Answer from the drawing. Dimensions are ordinates in mm from the lowest x, y and z of the part. Give positions to 0.01 mm unless a question says otherwise; leave off trailing zeros. Loops run counter-clockwise (first coordinate to the right, second up) from the corner with the lowest first, then second, coordinate; pieces in that order, holes last. Notation, with made-up numbers: (6.5, -12.5) - (31.5, -12.5) arc R28 ccw to (31.5, 7.5) - close; hole circle Ø8 at (75, 83.5). An arc over 180 degrees is marked (long way). Answer as CSV lines item,"result". Start each with the question number.
1) Find the intervals of material crossed by line 1 along Y through (x, z) = (0.6, 5) (1 decimal); line 2 along Z through (x, y) = (0.25, 4.25) (1 decimal); line 3 along Z through (x, y) = (0.1, 4.5) (1 decimal), in increasing order.
2) A cutting plane is placed at C-C (x = 0.1). Determine the outline of the cut face in (y, z) (1 decimal).
3) For a pull along Z with two mould halves and no side action, classify the marked faces 1, 2 and 3 as pulls with the +Z half, pulls with the -Z half, needs draft (parallel to the pull), parting line crosses it, or undercut.
4) A flat-ended cylindrical pin translates along its axis: pin 1 (1.9 mm diameter, centred on y = 3.96, z = 3.96, fed in from -X). Find the tip coordinate at first contact, or state that the pin passes through.
5) A cutting plane is placed at A-A (z = 4.75). Determine the outline of the cut face in (x, y) (1 decimal).
6) A cutting plane is placed at B-B (y = 4.5). Determine the outline of the cut face in (x, z).
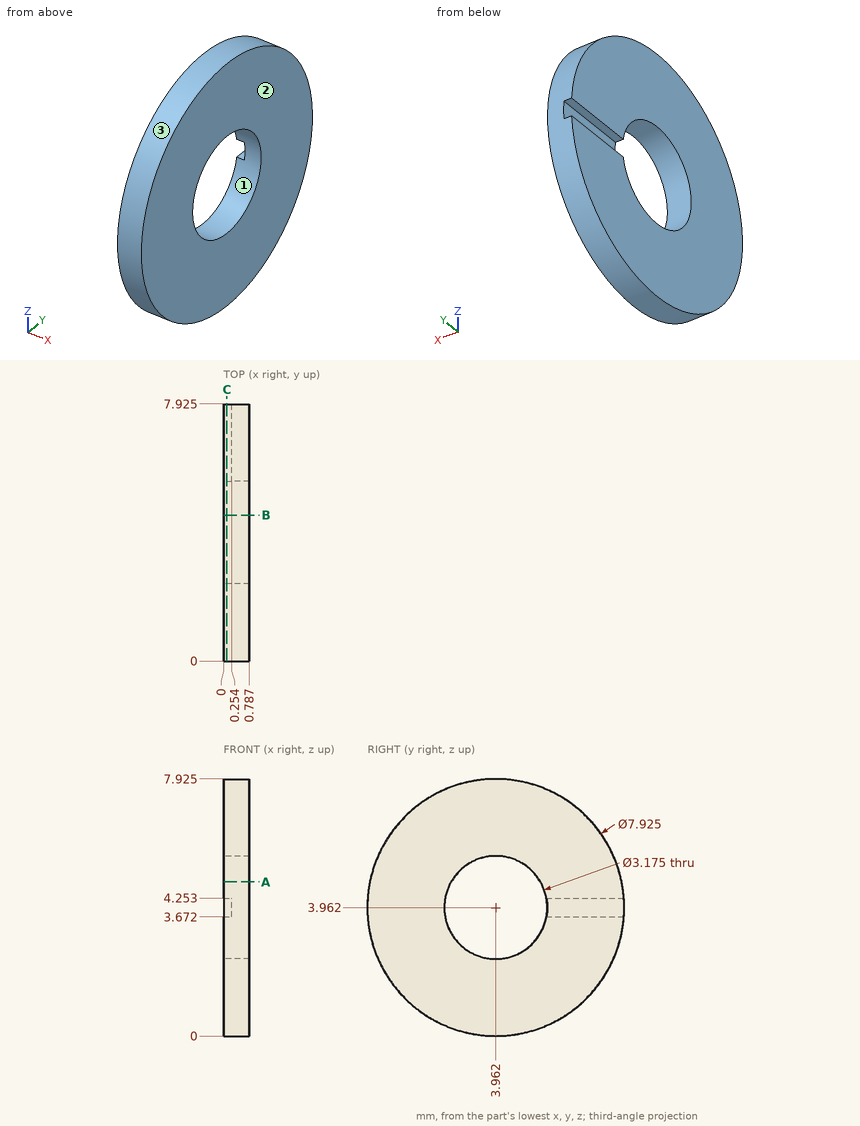
Ans:
1,line 1,"0.1 to 2.8, 5.2 to 7.8"
1,line 2,"0 to 2.4, 5.5 to 7.9"
1,line 3,"0 to 2.5, 5.5 to 7.9"
2,outline,"(5.5, 3.7) arc R1.6 cw (long way) to (5.5, 4.3) - (7.9, 4.3) arc R4 ccw (long way) to (7.9, 3.7) - close"
3,face 1,"undercut"
3,face 2,"needs draft"
3,face 3,"parting line crosses it"
4,pin 1,"through"
5,outline,"(0, 0.1) - (0.8, 0.1) - (0.8, 2.6) - (0, 2.6) - close; (0, 5.3) - (0.8, 5.3) - (0.8, 7.8) - (0, 7.8) - close"
6,outline,"(0, 0.04) - (0.79, 0.04) - (0.79, 2.47) - (0, 2.47) - close; (0, 5.46) - (0.79, 5.46) - (0.79, 7.89) - (0, 7.89) - close"
